Could you check a few things on this model? Use its own coordinates, in mm. A direction names the side the tool comes from. Coordinates: 2 decimals unless noted, no trailing zeros. Loops run counter-clockwise (first coordinate to the right, second up) from the corner with the lowest first, then second, coordinate; pieces in that order, holes last. Notation, with made-up numbers: (-1.5, 16) - (14.5, 16) arc R12 ccw to (14.5, 35) - close; hole circle Ø2 at (66.25, -2). An arc over 180 degrees is marked (long way). One line per item, written item: value. Start each with the question number.
(1) If we section it at C-C on y = 0.25: Write out the boundary of the cut face in (x, z).
(2) I'm going to push flat-ended pins straight in: P1, Ø0.5, axis at y = 2, z = 0.5, coming from the -X side; P2, Ø1.1, axis at x = -5.2, z = -2.54, coming from the -Y side; P3, Ø0.9, axis at x = 1.5, y = 2.5, coming from the +Z side; P4, Ø0.9, axis at y = 2, z = 0.5, coming from the +X side. Where does each tip first touch, or does it pass through?
(3) If we mould it in two halves opening along X, with no side actions, what happens to faces 5 (the face through (-4, 1.1, 0)), 6 (the face through (6.6, 0.5, 0.1)), 7 (the face through (-4.506, 0.558, -0.091)), 8 (the face through (-3.587, 2, 0))? For each: pulls with the +X half, pulls with the -X half, needs draft (parallel to the pull), parting line crosses it, or undercut.
(4) If I drill on line 1 along Z through (x, y) = (-5.25, 0.7); line 2 along X through (y, z) = (0.25, 0); line 3 along X through (y, z) = (2.1, -2.5), over which ranges is the centre line in solid material (lowest first)? Write a range as from..to.
(5) On a 3-axis mill with a long thin cutter (end or side, diameter ignored), from which of +Z, -Z, +X, -X, +Y, -Y can I reach the whole of each face in a straight line? I mean faces 1 (the face through (1, 2, -3.8)), 2 (the face through (6.213, 2, 0)), 3 (the face through (-4.6, 0.6, 2.9)), 4 (the face through (1, 2, 3.8)). Say none if no direction works.
(6) If we section it at B-B on x = -5.2: Write out the boundary of the cut face in (y, z).
(7) If we section it at D-D on z = -1.25: Write out the boundary of the cut face in (x, y), then the cut area to 3 significant figures.
(8) If we section it at A-A on z = 0: Write out the boundary of the cut face in (x, y), then the cut area to 3 significant figures.
```python
from build123d import *

# Parameters (mm, degrees)
SKETCH_1_W          = 13.2
SKETCH_1_H          = 8.2
EXTRUDE_1_DEPTH     = 1.1
SKETCH_3_W          = 9.8
SKETCH_3_H          = 7.6
EXTRUDE_2_DEPTH     = 1.8
SKETCH_2_R          = 0.7
CUT_EXTRUDE_1_DEPTH = 8.975587753


with BuildPart() as part:
    # Эскиз1 → Бобышка-Вытянуть1 (new body)
    with BuildSketch(Plane(origin=(0, 0, 0), x_dir=(1, 0, 0), z_dir=(0, 1, 0))):
        Rectangle(SKETCH_1_W, SKETCH_1_H)
    extrude(amount=EXTRUDE_1_DEPTH)

    # Эскиз3 → Бобышка-Вытянуть2 (add)
    with BuildSketch(Plane(origin=(0, 1.1, 0), x_dir=(1, 0, 0), z_dir=(0, 1, 0))):
        with Locations((1.313157895, 0)):
            Rectangle(SKETCH_3_W, SKETCH_3_H)
    extrude(amount=EXTRUDE_2_DEPTH)

    # Эскиз2 → Вырез-Вытянуть1 (cut, through all)
    with BuildSketch(Plane(origin=(0, 1.1, 0), x_dir=(1, 0, 0), z_dir=(0, 1, 0))):
        with Locations(Location((-5.2, -2.54, 0), (0, 0, 270))):
            Circle(SKETCH_2_R)
        with Locations(Location((-5.2, 0, 0), (0, 0, 270))):
            Circle(SKETCH_2_R)
        with Locations(Location((-5.2, 2.54, 0), (0, 0, 270))):
            Circle(SKETCH_2_R)
    extrude(amount=-CUT_EXTRUDE_1_DEPTH, mode=Mode.SUBTRACT)


solid = part.part
```
Values:
1. outline: (-6.6, -4.1) - (6.6, -4.1) - (6.6, 4.1) - (-6.6, 4.1) - close; hole circle Ø1.4 at (-5.2, -2.54); hole circle Ø1.4 at (-5.2, 0); hole circle Ø1.4 at (-5.2, 2.54)
2. P1: stops at x = -3.59
2. P2: passes through
2. P3: stops at z = 3.8
2. P4: stops at x = 6.21
3. face 5: needs draft
3. face 6: pulls with the +X half
3. face 7: undercut
3. face 8: pulls with the -X half
4. line 1: z = -4.1..-3.24, -1.84..-0.7, 0.7..1.84, 3.24..4.1
4. line 2: x = -6.6..-5.9, -4.5..6.6
4. line 3: x = -3.59..6.21
5. face 1: -Z, +X, -X, +Y
5. face 2: +Z, -Z, +X, +Y
5. face 3: +Y, -Y
5. face 4: +Z, +X, -X, +Y
6. outline: (0, -4.1) - (1.1, -4.1) - (1.1, -3.24) - (0, -3.24) - close; (0, -1.84) - (1.1, -1.84) - (1.1, -0.7) - (0, -0.7) - close; (0, 0.7) - (1.1, 0.7) - (1.1, 1.84) - (0, 1.84) - close; (0, 3.24) - (1.1, 3.24) - (1.1, 4.1) - (0, 4.1) - close
7. outline: (-6.6, 0) - (6.6, 0) - (6.6, 1.1) - (6.21, 1.1) - (6.21, 2.9) - (-3.59, 2.9) - (-3.59, 1.1) - (-6.6, 1.1) - close
7. area: 32.2 mm2
8. outline: (-6.6, 0) - (-5.9, 0) - (-5.9, 1.1) - (-6.6, 1.1) - close; (-4.5, 0) - (6.6, 0) - (6.6, 1.1) - (6.21, 1.1) - (6.21, 2.9) - (-3.59, 2.9) - (-3.59, 1.1) - (-4.5, 1.1) - close
8. area: 30.6 mm2
